```python
from build123d import *

# Parameters (mm, degrees)
BOSS_EXTRUDE3_DEPTH = 10
FILLET3_R           = 3


with BuildPart() as part:
    # Sketch1 → Boss-Extrude3 (new body)
    with BuildSketch(Plane(origin=(0, 0, 0), x_dir=(1, 0, 0), z_dir=(0, 1, 0))):
        with BuildLine():
            Line((-59.825295148, 15.68233951), (-56.816678559, 18.33423136))
            ThreePointArc((-56.816678559, 18.33423136), (-66.151990039, 22.514585376), (-75.433985922, 18.217149798))
            ThreePointArc((-75.433985922, 18.217149798), (-85.46391923, 10.174191538), (-75.433985922, 2.131233278))
            ThreePointArc((-75.433985922, 2.131233278), (-66.151990039, -2.1662023), (-56.816678559, 2.014151715))
            Line((-56.816678559, 2.014151715), (-59.825295148, 4.666043566))
            ThreePointArc((-59.825295148, 4.666043566), (-66.67551375, 1.865796025), (-73.051288265, 5.622973224))
            ThreePointArc((-73.051288265, 5.622973224), (-75.052192589, 6.694861395), (-77.224146609, 7.3545417))
            ThreePointArc((-77.224146609, 7.3545417), (-80.043796447, 10.174191538), (-77.224146609, 12.993841376))
            ThreePointArc((-77.224146609, 12.993841376), (-75.052192589, 13.653521681), (-73.051288265, 14.725409851))
            ThreePointArc((-73.051288265, 14.725409851), (-66.67551375, 18.48258705), (-59.825295148, 15.68233951))
        make_face()
    extrude(amount=BOSS_EXTRUDE3_DEPTH)

    # Fillet3
    fillet3_edges = [part.edges().sort_by_distance(p)[0] for p in [
        (-56.816678559, 5, -2.014151715),
        (-75.433985922, 5, -2.131233278),
        (-75.433985922, 5, -18.217149798),
        (-56.816678559, 5, -18.33423136),
    ]]
    fillet(fillet3_edges, radius=FILLET3_R)


solid = part.part
```
Input: part model. Units: mm. Frame: model coordinates. A direction names the side the tool comes from. Round coordinates to 2 decimals unless told otherwise and drop trailing zeros. Loops run counter-clockwise (first coordinate to the right, second up) from the corner with the lowest first, then second, coordinate; pieces in that order, holes last. Notation, with made-up numbers: (48.5, 8.25) - (71.5, 8.25) arc R18 ccw to (71.5, 40.25) - close; hole circle Ø6 at (71.25, 52.25). An arc over 180 degrees is marked (long way). One line per item, written item: value. Start each with the question number.
(1) Section B-B, the plane x = -61.75. Return loops of the section in (y, z), plus the area to 3 significant figures.
(2) Draft query along X for faces 3 (the flat face through (-75, 0, -5)), 4 (the cylindrical face through (-66.783, 4.93, -18.474)), 5 (the cylindrical face through (-66.57, 4.93, -1.86)), 6 (the cylindrical face through (-80.043, 4.93, -10.112)). Return one class per face: +X half, -X half, draft (parallel to the pull), parting line (faces both ways), or undercut.
(3) Section A-A, the plane z = -3.5. Return loops of the section in (x, y).
(4) Contact query for flat-ended pins moving along their axis: P1, Ø5, axis at x = -82.5, y = 8.5, coming from the +Z side; P2, Ø1.5, axis at x = -75, y = 7, coming from the +Z side; P3, Ø1, axis at y = 3, z = -12.5, coming from the -X side. Output: stop coordinate, or through.
(5) Section D-D, the plane z = -10. Return loops of the section in (x, y).
(6) Access query for faces 1 (the cylindrical face through (-67.595, 4.93, 2.072)), 2 (the cylindrical face through (-75.02, 4.93, -6.68)). Directions: +Z, -Z, +X, -X, +Y, -Y. A direction counts if a zero-diameter tool reaches every point of the face in a straight line with its end or side. Return the directions, or none.
(7) Ray query, line 1 (Z direction, x = -72, y = 5.25); line 2 (X direction, y = 2.25, z = -17.75); line 3 (Z direction, x = -72.5, y = 7). Return the intervals inside material, ascending. Write a range as [from, to].
(8) Section C-C, the plane x = -81.75. Return loops of the section in (y, z).
Results below:
1. outline: (0, -21.73) - (10, -21.73) - (10, -17.29) - (0, -17.29) - close; (0, -3.05) - (10, -3.05) - (10, 1.38) - (0, 1.38) - close
1. area: 88.8 mm^2
2. face 3: draft
2. face 4: undercut
2. face 5: undercut
2. face 6: +X half
3. outline: (-82.06, 0) - (-71.06, 0) - (-71.06, 10) - (-82.06, 10) - close; (-61.09, 0) - (-58.78, 0) - (-58.78, 10) - (-61.09, 10) - close
4. P1: z = -2.42
4. P2: z = -0.93
4. P3: x = -85.26
5. outline: (-85.46, 0) - (-80.04, 0) - (-80.04, 10) - (-85.46, 10) - close
6. face 1: +Z, +Y, -Y
6. face 2: +X, +Y, -Y
7. line 1: [-21, -16.03], [-4.32, 0.65]
7. line 2: [-80.46, -69.54], [-62.61, -58.47]
7. line 3: [-20.71, -15.48], [-4.87, 0.36]
8. outline: (0, -17.06) - (10, -17.06) - (10, -3.29) - (0, -3.29) - close
